```python
from build123d import *

# Parameters (mm, degrees)
SKETCH1_W           = 24
SKETCH1_H           = 16
SKETCH1_R           = 1.65
BOSS_EXTRUDE1_DEPTH = 4.8
SKETCH2_W           = 3
SKETCH2_H           = 2.8
BOSS_EXTRUDE2_DEPTH = 70
SKETCH4_W           = 6.5
SKETCH4_H           = 21.5
BOSS_EXTRUDE3_DEPTH = 4.8


with BuildPart() as part:
    # Sketch1 → Boss-Extrude1 (new body)
    with BuildSketch(Plane.XZ):
        with Locations((12, -8)):
            Rectangle(SKETCH1_W, SKETCH1_H)
        with Locations((8, -8)):
            Circle(SKETCH1_R, mode=Mode.SUBTRACT)
        with Locations((16, -8)):
            Circle(SKETCH1_R, mode=Mode.SUBTRACT)
    extrude(amount=BOSS_EXTRUDE1_DEPTH)

    # Sketch2 → Boss-Extrude2 (add)
    with BuildSketch(Plane.XY):
        with Locations((7.5, -1.4)):
            Rectangle(SKETCH2_W, SKETCH2_H)
        with Locations((16.5, -1.4)):
            Rectangle(SKETCH2_W, SKETCH2_H)
    extrude(amount=BOSS_EXTRUDE2_DEPTH)

    # Sketch4 → Boss-Extrude3 (add)
    with BuildSketch(Plane(origin=(0, 0, 0), x_dir=(1, 0, 0), z_dir=(0, 1, 0))):
        with Locations((3.25, 26.75)):
            Rectangle(SKETCH4_W, SKETCH4_H)
    extrude(amount=-BOSS_EXTRUDE3_DEPTH)


solid = part.part
```
Can you work these out from the model? Positions are in its coordinate system, mm. A direction names the side the tool comes from. Round coordinates to 2 decimals unless told otherwise and drop trailing zeros. Loops run counter-clockwise (first coordinate to the right, second up) from the corner with the lowest first, then second, coordinate; pieces in that order, holes last. Notation, with made-up numbers: (81.5, 64) -> (107.5, 64) arc R15 ccw to (107.5, 81) -> close; hole circle Ø6 at (38, -38.5). An arc over 180 degrees is marked (long way). Answer in a Markdown table with one row per item.
Item 1: Will these pins go through, and if not, where does the flat tip stop? P1, Ø6, axis at x = 19.5, z = 31.5, coming from the -Y side; P2, Ø0.8, axis at y = -1, z = 32, coming from the +X side; P3, Ø1.4, axis at y = -1, z = 31.5, coming from the -X side.
Answer block:
| item | result |
|---|---|
| P1 | y = -2.8 |
| P2 | x = 18 |
| P3 | x = 6 |
Item 2: Suppose I cut it at D-D, the plane x = 22. List the corners of the cut face in (y, z) for me.
Answer block:
| item | result |
|---|---|
| outline | (-4.8, -16) -> (0, -16) -> (0, 0) -> (-4.8, 0) -> close |
Item 3: We'd pull the mould along X, two halves only. Please class faces 1 (the flat face through (16, -2.8, 35)), 2 (the flat face through (12, -2, 0)), 3 (the flat face through (24, -2, -8)), 4 (the cylindrical face through (6.69, -2.37, -9)): released by +X, released by -X, zero draft, split by the parting line, or undercut.
Answer block:
| item | result |
|---|---|
| face 1 | zero draft |
| face 2 | undercut |
| face 3 | released by +X |
| face 4 | undercut |
Item 4: Suppose I cut it at C-C, the plane x = 8. List the corners of the cut face in (y, z) for me.
Answer block:
| item | result |
|---|---|
| outline | (-4.8, -16) -> (0, -16) -> (0, -9.65) -> (-4.8, -9.65) -> close; (-4.8, -6.35) -> (0, -6.35) -> (0, 70) -> (-2.8, 70) -> (-2.8, 0) -> (-4.8, 0) -> close |
Item 5: Suppose I cut it at B-B, the plane y = -2. List the corners of the cut face in (x, z) for me.
Answer block:
| item | result |
|---|---|
| outline | (0, -37.5) -> (6.5, -37.5) -> (6.5, -16) -> (24, -16) -> (24, 0) -> (18, 0) -> (18, 70) -> (15, 70) -> (15, 0) -> (9, 0) -> (9, 70) -> (6, 70) -> (6, 0) -> (0, 0) -> close; hole circle Ø3.3 at (8, -8); hole circle Ø3.3 at (16, -8) |
Item 6: On a 3-axis mill with a long thin cutter (end or side, diameter ignored), from which of +Z, -Z, +X, -X, +Y, -Y can I reach the whole of each face in a straight line? I mean faces 5 (the flat face through (6.5, -2, -27)), 6 (the flat face through (6, -1, 35)), 7 (the flat face through (15, -1, 35)), 8 (the flat face through (18, -1, 35)), 9 (the flat face through (7, -2.8, 35)). Say none if no direction works.
Answer block:
| item | result |
|---|---|
| face 5 | -Z, +X, +Y, -Y |
| face 6 | +Z, -X, +Y, -Y |
| face 7 | +Z, +Y, -Y |
| face 8 | +Z, +X, +Y, -Y |
| face 9 | +Z, +X, -X, -Y |
Item 7: If I drill on probe 1 along X at (y, z) = (-1.5, 34.5); probe 2 along Z at (x, y) = (16, -3.75); probe 3 along Z at (x, y) = (16, -1.15), over which ranges is the centre line in solid material (lowest first)?
Answer block:
| item | result |
|---|---|
| probe 1 | 6 to 9, 15 to 18 |
| probe 2 | -16 to -9.65, -6.35 to 0 |
| probe 3 | -16 to -9.65, -6.35 to 70 |
Item 8: Suppose I cut it at A-A, the plane z = -8. List the corners of the cut face in (x, y) for me, plus the area to 3 significant figures.
Answer block:
| item | result |
|---|---|
| outline | (0, -4.8) -> (6.35, -4.8) -> (6.35, 0) -> (0, 0) -> close; (9.65, -4.8) -> (14.35, -4.8) -> (14.35, 0) -> (9.65, 0) -> close; (17.65, -4.8) -> (24, -4.8) -> (24, 0) -> (17.65, 0) -> close |
| area | 83.5 mm² |
